```python
from build123d import *

# Parameters (mm, degrees)
F0_W      = 78.334294
F0_H      = 72.097283
F1_DEPTH  = 76.2
F2_R      = 18.111105
F3_DEPTH  = 33.02
F4_R      = 6.35
F5_DEPTH  = 50.8
F6_R      = 12.471765
F7_DEPTH  = 33.02
F8_R      = 23.903657
F9_DEPTH  = 17.78
F10_R     = 30.618362
F11_DEPTH = 10.16


with BuildPart() as f1:
    # F0 (on Top) → F1 (new body)
    with BuildSketch(Plane.XY):
        with Locations((2.11006, 3.617437)):
            Rectangle(F0_W, F0_H)
    extrude(amount=F1_DEPTH)

    # F2 (on face) → F3 (cut)
    with BuildSketch(Plane.XY.offset(76.2)):
        Circle(F2_R)
    extrude(amount=-F3_DEPTH, mode=Mode.SUBTRACT)

    # F4 (on face) → F5 (cut)
    with BuildSketch(Plane.XY.offset(43.18)):
        Circle(F4_R)
    extrude(amount=-F5_DEPTH, mode=Mode.SUBTRACT)

    # F6 (on face) → F7 (cut)
    with BuildSketch(Plane.XY.offset(43.18)):
        Circle(F6_R)
    extrude(amount=-F7_DEPTH, mode=Mode.SUBTRACT)

    # F8 (on face) → F9 (cut)
    with BuildSketch(Plane.XY.offset(76.2)):
        Circle(F8_R)
    extrude(amount=-F9_DEPTH, mode=Mode.SUBTRACT)

    # F10 (on face) → F11 (cut)
    with BuildSketch(Plane.XY.offset(76.2)):
        Circle(F10_R)
    extrude(amount=-F11_DEPTH, mode=Mode.SUBTRACT)


solid = f1.part
```
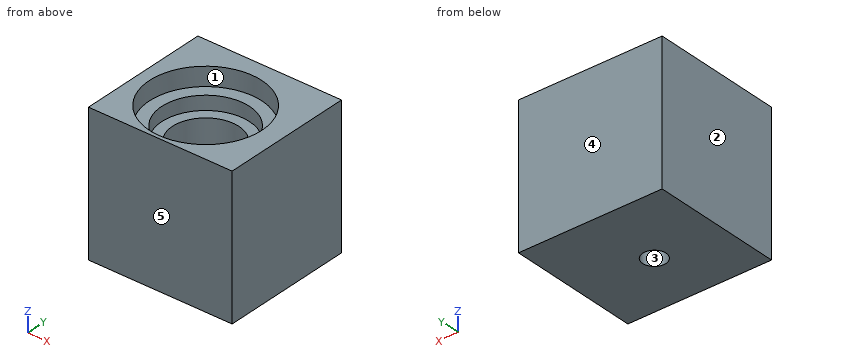
Geometry check sheet. Reference: the model listing, model coordinates, mm. Face numbers are marked on the shaded views. A direction names the side the tool comes from. Round coordinates to 2 decimals unless told otherwise and drop trailing zeros. Loops run counter-clockwise (first coordinate to the right, second up) from the corner with the lowest first, then second, coordinate; pieces in that order, holes last. Notation, with made-up numbers: M 15.5,77.25 L 48.5,77.25 A11 cw 48.5,88.25 Z; hole C 74.5,9.25 d5. An arc over 180 degrees is marked long. Return JSON: item names as keys, results as strings. Group by question number.
(1) Section check C-C, the plane z = 39.5. Enter the section's corners in (x, y), and give its area (3 significant figures).
(2) Section check D-D, the plane x = 26. Enter the section's corners in (y, z).
(3) Go/stop test with flat-tipped pins: pin 1 (7.5 mm diameter, centred on x = 0.5, y = -6, fed in from +Z); pin 2 (11.5 mm diameter, centred on x = 0, y = 0, fed in from +Z); pin 3 (4 mm diameter, centred on x = -12, y = 11.5, fed in from +Z). Record where each tip stops, or that it passes through.
(4) Section check A-A, the plane x = 0. Enter the section's corners in (y, z).
(5) Scan lines: line 1 along Y through (x, z) = (0, 36); line 2 along Y through (x, z) = (0, 6.25); line 3 along Z through (x, y) = (7, 18). Record each from-to range of solid material in increasing order. Write a range as [from, to].
(6) Set-up check for the marked faces 1 and 2: record each of +Z, -Z, +X, -X, +Y, -Y from which the full face is reachable in a straight line by a thin tool's end or side.
(7) Section check B-B, the plane y = 0. Enter the section's corners in (x, z), and give its area (3 significant figures).
(8) Mould release check, pull along Y, two halves, no side actions. Record for the marked faces 3, 4 and 5: pulls with the +Y half, pulls with the -Y half, needs draft (parallel to the pull), parting line crosses it, or undercut.
Data:
{
 "1": {"outline": "M -37.06,-32.43 L 41.28,-32.43 L 41.28,39.67 L -37.06,39.67 Z; hole C 0,0 d24.94", "area": "5,160 mm²"},
 "2": {"outline": "M -32.43,0 L 39.67,0 L 39.67,76.2 L 16.17,76.2 L 16.17,66.04 L -16.17,66.04 L -16.17,76.2 L -32.43,76.2 Z"},
 "3": {"pin 1": "z = 10.16", "pin 2": "through", "pin 3": "z = 58.42"},
 "4": {"outline": "M -32.43,0 L -6.35,0 L -6.35,10.16 L -12.47,10.16 L -12.47,43.18 L -18.11,43.18 L -18.11,58.42 L -23.9,58.42 L -23.9,66.04 L -30.62,66.04 L -30.62,76.2 L -32.43,76.2 Z; M 6.35,0 L 39.67,0 L 39.67,76.2 L 30.62,76.2 L 30.62,66.04 L 23.9,66.04 L 23.9,58.42 L 18.11,58.42 L 18.11,43.18 L 12.47,43.18 L 12.47,10.16 L 6.35,10.16 Z"},
 "5": {"line 1": "[-32.43, -12.47], [12.47, 39.67]", "line 2": "[-32.43, -6.35], [6.35, 39.67]", "line 3": "[0, 58.42]"},
 "6": {"face 1": "+Z", "face 2": "+Z, -Z, -X, +Y, -Y"},
 "7": {"outline": "M -37.06,0 L -6.35,0 L -6.35,10.16 L -12.47,10.16 L -12.47,43.18 L -18.11,43.18 L -18.11,58.42 L -23.9,58.42 L -23.9,66.04 L -30.62,66.04 L -30.62,76.2 L -37.06,76.2 Z; M 6.35,0 L 41.28,0 L 41.28,76.2 L 30.62,76.2 L 30.62,66.04 L 23.9,66.04 L 23.9,58.42 L 18.11,58.42 L 18.11,43.18 L 12.47,43.18 L 12.47,10.16 L 6.35,10.16 Z", "area": "3,480 mm²"},
 "8": {"face 3": "undercut", "face 4": "pulls with the +Y half", "face 5": "pulls with the -Y half"}
}
